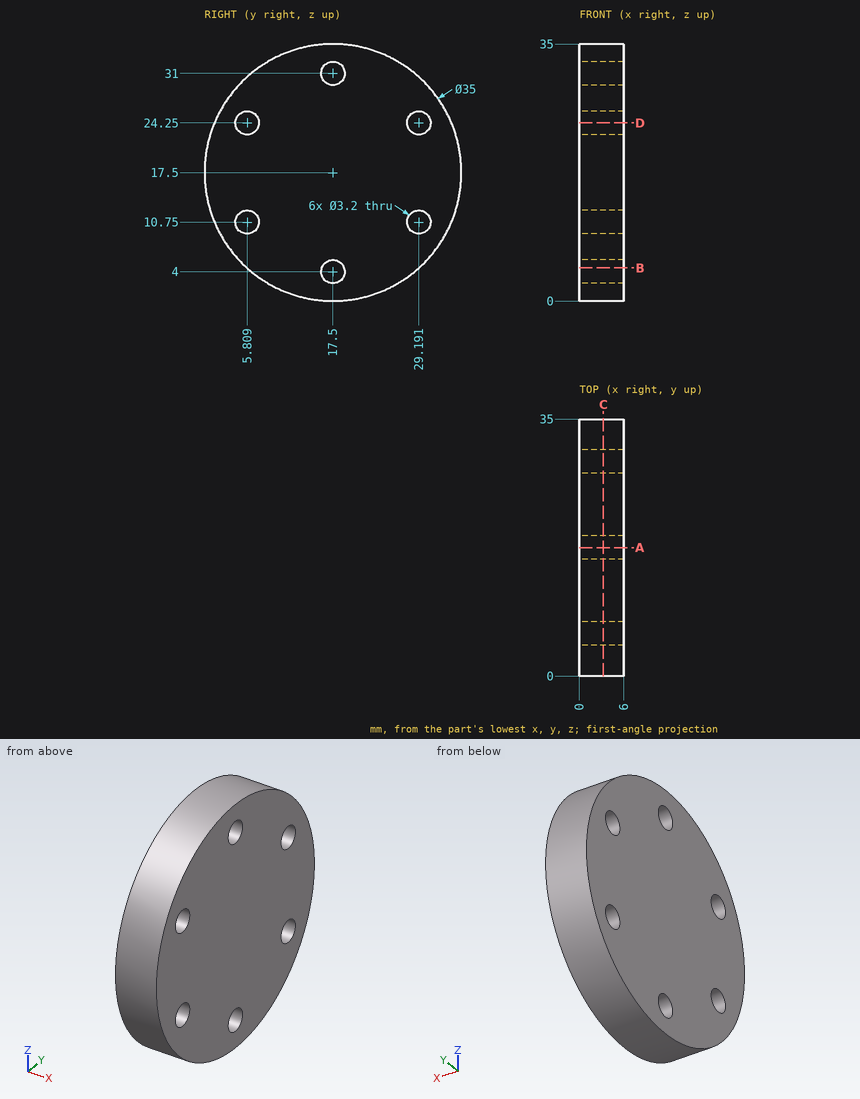
The drawing under review shows one solid part. Ordinate dimensions are in mm from its lowest x, y, z. Coordinates: 2 decimals unless noted, no trailing zeros. Write each loop counter-clockwise with the first axis right and the second up, starting at its lowest first coordinate (ties: lowest second). Pieces come first, ordered by that corner, then holes. Notation, with made-up numbers: (1, -37) -> (49, -37) arc R15 ccw to (49, -18) -> close; hole circle Ø1 at (81, -27). An arc over 180 degrees is marked (long way). Write each question's results on one line, items separated by ' | '. Start each with the question number.
1) Consider section D-D (z = 24.25). Write out the cut boundary in (x, y).
2) Consider section C-C (x = 3.25). Write out the cut boundary in (y, z).
3) Consider section B-B (z = 4.5). Write out the cut boundary in (x, y) (1 decimal), plus the area to 3 significant figures.
4) Insertion check: pin 1 (2 mm diameter, centred on x = 2.5, z = 28, fed in from +Y); pin 2 (2.5 mm diameter, centred on y = 29.19, z = 10.75, fed in from +X); pin 3 (1 mm diameter, centred on x = 4, y = 28.5, fed in from +Z). Each pin has a flat end and moves straight along its axis. Give the tip position at first contact, or say it passes through.
5) Consider section A-A (y = 17.5). Write out the cut boundary in (x, z), plus the area to 3 significant figures.
6) Wall thickness on L1, parallel to Z at x = 3.9, y = 17.5; L2, parallel to Y at x = 2.65, z = 12 (1 decimal); L3, parallel to Y at x = 4.6, z = 24.25 (1 decimal): over which ranges is each line inside the solid? List them lowest first. Write a range as [from, to].
Geometry says:
1) outline: (0, 1.35) -> (6, 1.35) -> (6, 4.21) -> (0, 4.21) -> close; (0, 7.41) -> (6, 7.41) -> (6, 27.59) -> (0, 27.59) -> close; (0, 30.79) -> (6, 30.79) -> (6, 33.65) -> (0, 33.65) -> close
2) outline: circle Ø35 at (17.5, 17.5); hole circle Ø3.2 at (5.81, 10.75); hole circle Ø3.2 at (5.81, 24.25); hole circle Ø3.2 at (17.5, 4); hole circle Ø3.2 at (17.5, 31); hole circle Ø3.2 at (29.19, 10.75); hole circle Ø3.2 at (29.19, 24.25)
3) outline: (0, 5.8) -> (6, 5.8) -> (6, 16) -> (0, 16) -> close; (0, 19) -> (6, 19) -> (6, 29.2) -> (0, 29.2) -> close | area: 122 mm^2
4) pin 1: y = 32.2 | pin 2: through | pin 3: z = 31.5
5) outline: (0, 0) -> (6, 0) -> (6, 2.4) -> (0, 2.4) -> close; (0, 5.6) -> (6, 5.6) -> (6, 29.4) -> (0, 29.4) -> close; (0, 32.6) -> (6, 32.6) -> (6, 35) -> (0, 35) -> close | area: 172 mm^2
6) L1: [0, 2.4], [5.6, 29.4], [32.6, 35] | L2: [0.9, 4.8], [6.8, 28.2], [30.2, 34.1] | L3: [1.4, 4.2], [7.4, 27.6], [30.8, 33.6]
